Could you check a few things on this model? Use its own coordinates, in mm. A direction names the side the tool comes from. Give positions to 0.01 mm unless a question says otherwise; leave off trailing zeros. Loops run counter-clockwise (first coordinate to the right, second up) from the corner with the lowest first, then second, coordinate; pieces in that order, holes last. Notation, with made-up numbers: (-17, 38.25) - (35, 38.25) arc R24 cw to (35, 66.25) - close; hole circle Ø8 at (60, 36). An arc over 180 degrees is marked (long way). Write each question's results on one line, items separated by ' | '. Start each with the question number.
(1) If we mould it in two halves opening along X, with no side actions, what happens to faces 1 (the face through (81, 62.075, 1)), 2 (the face through (50.23, 39.41, 1.52)), 3 (the face through (-3, 58, 1))? For each: released by +X, released by -X, zero draft, split by the parting line, or undercut.
(2) Suppose I cut it at B-B (y = 0). Please give me the cut outline in (x, z).
(3) Suppose I cut it at A-A (x = 42.5). Please give me the cut outline in (y, z).
(4) I need wall thicknesses on line 1 (X direction, y = 22.5, z = 1.85); line 2 (Y direction, x = 19, z = 0.7); line 3 (X direction, y = 44.5, z = 2.25). Which ranges of each line are inside material? Lowest first, please.
(5) Suppose I cut it at C-C (x = 28.5). Please give me the cut outline in (y, z), and give its area (3 significant figures).
(6) For pin 1 (1 mm diameter, centred on y = 32, z = 2, fed in from -X); pin 2 (0.9 mm diameter, centred on x = 60.5, z = 1.5, fed in from -Y); pin 3 (0.8 mm diameter, centred on y = 50, z = 2, fed in from +X); pin 4 (12 mm diameter, centred on x = 18.5, y = 32.5, fed in from -Z), each with a flat end and sliding along its axis, tell me the tip position at first contact or that it passes through.
(7) Suppose I cut it at D-D (z = 1.8). Count the separate pieces of the cut face and the enclosed holes in it, and give its area (3 significant figures).
(8) On a 3-axis mill with a long thin cutter (end or side, diameter ignored), from which of +Z, -Z, +X, -X, +Y, -Y can I reach the whole of each face in a straight line? I mean faces 4 (the face through (60, 20.8, 1)), 5 (the face through (40, 7.5, 1)), 6 (the face through (39, 31, 3)), 7 (the face through (81, 40.925, 1)). Say none if no direction works.
from build123d import *

# Parameters (mm, degrees)
SKETCH_1_R          = 1.65
EXTRUDE_1_DEPTH     = 3
FILLET_1_R          = 5
CUT_EXTRUDE_1_DEPTH = 111.550893257
FILLET_2_R          = 1


with BuildPart() as part:
    # 草图1 → 凸台-拉伸1 (new body)
    with BuildSketch(Plane.XY):
        with BuildLine():
            Line((7.014012459, -2.655866944), (10.859547587, 7.5))
            Line((10.859547587, 7.5), (69.140452413, 7.5))
            Line((69.140452413, 7.5), (72.985987541, -2.655866944))
            ThreePointArc((72.985987541, -2.655866944), (82.655866944, -7.014012459), (87.014012459, 2.655866944))
            Line((87.014012459, 2.655866944), (79.5, 22.5))
            Line((79.5, 22.5), (79.5, 32.925))
            Line((79.5, 32.925), (83, 32.925))
            Line((83, 32.925), (83, 40.925))
            Line((83, 40.925), (79.5, 40.925))
            Line((79.5, 40.925), (79.5, 54.075))
            Line((79.5, 54.075), (83, 54.075))
            Line((83, 54.075), (83, 62.075))
            Line((83, 62.075), (79.5, 62.075))
            Line((79.5, 62.075), (79.5, 67.5))
            Line((79.5, 67.5), (0.5, 67.5))
            Line((0.5, 67.5), (0.5, 62.075))
            Line((0.5, 62.075), (-3, 62.075))
            Line((-3, 62.075), (-3, 54.075))
            Line((-3, 54.075), (0.5, 54.075))
            Line((0.5, 54.075), (0.5, 40.925))
            Line((0.5, 40.925), (-3, 40.925))
            Line((-3, 40.925), (-3, 32.925))
            Line((-3, 32.925), (0.5, 32.925))
            Line((0.5, 32.925), (0.5, 22.5))
            Line((0.5, 22.5), (-7.014012459, 2.655866944))
            ThreePointArc((-7.014012459, 2.655866944), (-2.655866944, -7.014012459), (7.014012459, -2.655866944))
        make_face()
        Circle(SKETCH_1_R, mode=Mode.SUBTRACT)
        with Locations((80, 0)):
            Circle(SKETCH_1_R, mode=Mode.SUBTRACT)
        with BuildLine():
            Line((15, 24.2), (25, 24.2))
            ThreePointArc((25, 24.2), (26.7, 22.5), (25, 20.8))
            Line((25, 20.8), (15, 20.8))
            ThreePointArc((15, 20.8), (13.3, 22.5), (15, 24.2))
        make_face(mode=Mode.SUBTRACT)
        with BuildLine():
            Line((65, 24.2), (55, 24.2))
            ThreePointArc((55, 24.2), (53.3, 22.5), (55, 20.8))
            Line((55, 20.8), (65, 20.8))
            ThreePointArc((65, 20.8), (66.7, 22.5), (65, 24.2))
        make_face(mode=Mode.SUBTRACT)
    extrude(amount=EXTRUDE_1_DEPTH)

    # 圆角1
    fillet_1_edges = [part.edges().sort_by_distance(p)[0] for p in [
        (69.140452413, 7.5, 1.5),
        (10.859547587, 7.5, 1.5),
        (0.5, 67.5, 1.5),
        (79.5, 67.5, 1.5),
    ]]
    fillet(fillet_1_edges, radius=FILLET_1_R)

    # 草图3 → 切除-拉伸1 (cut, through all)
    with BuildSketch(Plane.XY.offset(3)):
        Polygon((0.5, 45.8), (4, 45.8), (4, 44.25), (7.5, 44.25), (7.5, 45.8), (10.9, 45.8), (10.9, 49.2), (7.5, 49.2), (7.5, 50.75), (4, 50.75), (4, 49.2), (0.5, 49.2), align=None)
        Polygon((79.5, 49.2), (76, 49.2), (76, 50.75), (72.5, 50.75), (72.5, 49.2), (69.1, 49.2), (69.1, 45.8), (72.5, 45.8), (72.5, 44.25), (76, 44.25), (76, 45.8), (79.5, 45.8), align=None)
        Polygon((40, 51.5), (15, 61.5), (65, 61.5), align=None)
        Polygon((65, 33.5), (40, 43.5), (15, 33.5), align=None)
    extrude(amount=-CUT_EXTRUDE_1_DEPTH, mode=Mode.SUBTRACT)

    # 圆角2
    fillet_2_edges = [part.edges().sort_by_distance(p)[0] for p in [
        (65, 61.5, 1.5),
        (15, 61.5, 1.5),
        (65, 33.5, 1.5),
        (15, 33.5, 1.5),
    ]]
    fillet(fillet_2_edges, radius=FILLET_2_R)


solid = part.part
Output values:
1) face 1: zero draft | face 2: undercut | face 3: released by -X
2) outline: (-7.5, 0) - (-1.65, 0) - (-1.65, 3) - (-7.5, 3) - close; (1.65, 0) - (8.02, 0) - (8.02, 3) - (1.65, 3) - close; (71.98, 0) - (78.35, 0) - (78.35, 3) - (71.98, 3) - close; (81.65, 0) - (87.5, 0) - (87.5, 3) - (81.65, 3) - close
3) outline: (7.5, 0) - (33.5, 0) - (33.5, 3) - (7.5, 3) - close; (42.5, 0) - (52.5, 0) - (52.5, 3) - (42.5, 3) - close; (61.5, 0) - (67.5, 0) - (67.5, 3) - (61.5, 3) - close
4) line 1: 0.5 to 13.3, 26.7 to 53.3, 66.7 to 79.5 | line 2: 7.5 to 20.8, 24.2 to 67.5 | line 3: 0.5 to 4, 7.5 to 72.5, 76 to 79.5
5) outline: (7.5, 0) - (33.5, 0) - (33.5, 3) - (7.5, 3) - close; (38.9, 0) - (56.1, 0) - (56.1, 3) - (38.9, 3) - close; (61.5, 0) - (67.5, 0) - (67.5, 3) - (61.5, 3) - close | area: 148 mm2
6) pin 1: x = 0.5 | pin 2: y = 7.5 | pin 3: x = 79.5 | pin 4: z = 0
7) separate pieces: 1 | enclosed holes: 6 | area: 4,670 mm2
8) face 4: +Z, -Z | face 5: +Z, -Z, -Y | face 6: +Z, +X, -X, +Y, -Y | face 7: +Z, -Z, +X
